The listing builds one solid part. Answer for the finished solid, in the listing's coordinates (mm). Face numbers are marked on the shaded views. A direction names the side the tool comes from. Coordinates: 2 decimals unless noted, no trailing zeros. Write each loop counter-clockwise with the first axis right and the second up, starting at its lowest first coordinate (ties: lowest second). Pieces come first, ordered by that corner, then holes.
(1) The part is cut by section B-B on y = 11. Determine the outline of the cut face in (x, z), plus the area to 3 significant figures.
(2) Which of the six approach directions +Z, -Z, +X, -X, +Y, -Y give full straight-line access (tool end or side, diameter ignored) to the marked faces 1 and 2?
(3) The part is cut by section A-A on z = -0.5. Determine the outline of the cut face in (x, y), plus the area to 3 significant figures.
(4) The part is cut by section D-D on y = 2. Determine the outline of the cut face in (x, z).
(5) Straight lines are drawn through the part: line 1 (X direction, y = 20, z = -6); line 2 (Z direction, x = -2.75, y = 27.5); line 3 (Z direction, x = -19.5, y = 32.5). For each, find the intervals that lie inside material, in ascending order.
(6) For a pull along X with two mould halves and no side action, classify the marked faces 3, 4 and 5 as +X half, -X half, draft (parallel to the pull), parting line (faces both ways), or undercut.
(7) The part is cut by section C-C on x = -1.75. Determine the outline of the cut face in (y, z).
(8) Given P1, Ø1.7, axis at x = -22, y = 20, coming from the +Z side; P2, Ø4, axis at x = -10, z = -12, coming from the -Y side; P3, Ø0.8, axis at x = -2, y = 2, coming from the +Z side, each flat-ended and moving along its own axis, determine where each tip first touches the part or whether it passes through.
from build123d import *

# Parameters (mm, degrees)
PROFILE_EXTRUDE_DEPTH  = 40
SPROCKET_SKETCH_R      = 0.75
SPROCKET_EXTRUDE_DEPTH = 1


with BuildPart() as part:
    # Profile Sketch → Profile Extrude (new body)
    with BuildSketch(Plane(origin=(0.045617437, 0, -0.024209872), x_dir=(-1, 0, 0), z_dir=(0, 1, 0))):
        Polygon((5.945617437, -11.975790128), (5.945617437, 0.024209872), (-0.054382563, 0.024209872), (-0.054382563, 2.024209872), (-0.954382563, 2.024209872), (-0.954382563, -14.475790128), (25.045617437, -14.475790128), (25.045617437, 2.024209872), (24.145617437, 2.024209872), (24.145617437, 0.024209872), (20.795617437, 0.024209872), (20.795617437, -11.975790128), align=None)
    extrude(amount=PROFILE_EXTRUDE_DEPTH)

    # Sprocket Sketch → Sprocket Extrude (add)
    with BuildSketch(Plane.XY):
        with Locations(Location((-1.75, 2, 0), (0, 0, 180))):
            Circle(SPROCKET_SKETCH_R)
    extrude(amount=SPROCKET_EXTRUDE_DEPTH)


solid = part.part
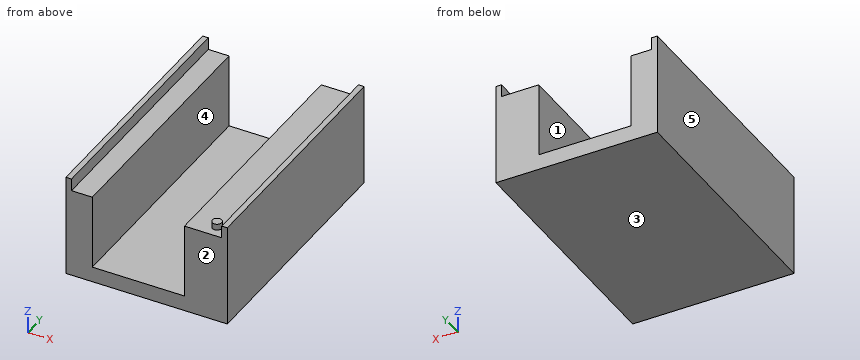
Model answer:
1. outline: (-25, -14.5) - (1, -14.5) - (1, 2) - (0.1, 2) - (0.1, 0) - (-5.9, 0) - (-5.9, -12) - (-20.75, -12) - (-20.75, 0) - (-24.1, 0) - (-24.1, 2) - (-25, 2) - close
1. area: 202 mm2
2. face 1: +Z, +Y, -Y
2. face 2: +Z, -Z, +X, -X, -Y
3. outline: (-25, 0) - (-20.75, 0) - (-20.75, 40) - (-25, 40) - close; (-5.9, 0) - (1, 0) - (1, 40) - (-5.9, 40) - close
3. area: 446 mm2
4. outline: (-25, -14.5) - (1, -14.5) - (1, 2) - (0.1, 2) - (0.1, 0) - (-1, 0) - (-1, 1) - (-2.5, 1) - (-2.5, 0) - (-5.9, 0) - (-5.9, -12) - (-20.75, -12) - (-20.75, 0) - (-24.1, 0) - (-24.1, 2) - (-25, 2) - close
5. line 1: x = -25 to -20.75, -5.9 to 1
5. line 2: z = -14.5 to 0
5. line 3: z = -14.5 to -12
6. face 3: draft
6. face 4: undercut
6. face 5: -X half
7. outline: (0, -14.5) - (40, -14.5) - (40, 0) - (2.75, 0) - (2.75, 1) - (1.25, 1) - (1.25, 0) - (0, 0) - close
8. P1: stops at z = 0
8. P2: stops at y = 0
8. P3: stops at z = 1
